```python
from build123d import *

# Parameters (mm, degrees)
SKETCH1_W           = 14
SKETCH1_H           = 10
SKETCH1_W_2         = 30
SKETCH1_H_2         = 30
BOSS_EXTRUDE1_DEPTH = 10
FILLET1_R           = 2


with BuildPart() as part:
    # Sketch1 → Boss-Extrude1 (new body)
    with BuildSketch(Plane.XY):
        with Locations((0, -5)):
            Rectangle(SKETCH1_W, SKETCH1_H)
        with Locations((0, 15)):
            Rectangle(SKETCH1_W_2, SKETCH1_H_2)
    extrude(amount=BOSS_EXTRUDE1_DEPTH)

    # Fillet1
    fillet1_edges = [part.edges().sort_by_distance(p)[0] for p in [
        (7, -10, 5),
        (-7, -10, 5),
        (-15, 0, 5),
        (-15, 30, 5),
        (15, 30, 5),
        (15, 0, 5),
    ]]
    fillet(fillet1_edges, radius=FILLET1_R)


solid = part.part
```
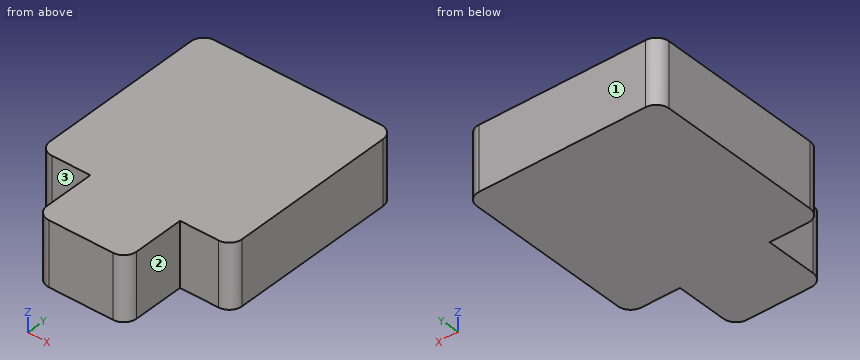
Check sheet for the modelled part. Datum: model origin and axes. Units: mm. Face numbers are marked on the shaded views. A direction names the side the tool comes from. Give positions to 0.01 mm unless a question says otherwise; leave off trailing zeros. Loops run counter-clockwise (first coordinate to the right, second up) from the corner with the lowest first, then second, coordinate; pieces in that order, holes last. Notation, with made-up numbers: (-15, 60.25) - (11, 60.25) arc R24 cw to (11, 70.25) - close; hole circle Ø3 at (4, 22). An arc over 180 degrees is marked (long way). One line per question, with ' | ' between items. Start each with the question number.
1. Gauge pin test, flat ends, axial feed: pin 1 Ø3 at (x, z) = (-9, 4) entering from -Y; pin 2 Ø6 at (x, y) = (-10.5, 14) entering from -Z; pin 3 Ø1.5 at (y, z) = (-2.5, 5) entering from -X; pin 4 Ø2.5 at (y, z) = (-5.5, 3) entering from +X. Record the tip position at first contact, or that the pin passes through.
2. Cross-section at B-B, the plane y = -4.5. Enter the section's corners in (x, z), plus the area to 3 significant figures.
3. Material ranges on line 1 along Y through (x, z) = (7.5, 6.5); line 2 along X through (y, z) = (-6, 3.5); line 3 along Y through (x, z) = (-6.75, 3.75), recorded low to high. Write a range as [from, to].
4. Cross-section at C-C, the plane x = 8.25. Enter the section's corners in (y, z).
5. Cross-section at A-A, the plane z = 4. Enter the section's corners in (x, y), plus the area to 3 significant figures.
6. Set-up check for the marked faces 1, 2 and 3: record each of +Z, -Z, +X, -X, +Y, -Y from which the full face is reachable in a straight line by a thin tool's end or side.
Check result:
1) pin 1: stops at y = 0 | pin 2: stops at z = 0 | pin 3: stops at x = -7 | pin 4: stops at x = 7
2) outline: (-7, 0) - (7, 0) - (7, 10) - (-7, 10) - close | area: 140 mm2
3) line 1: y = [0, 30] | line 2: x = [-7, 7] | line 3: y = [-8.97, 30]
4) outline: (0, 0) - (30, 0) - (30, 10) - (0, 10) - close
5) outline: (-15, 2) arc R2 ccw to (-13, 0) - (-7, 0) - (-7, -8) arc R2 ccw to (-5, -10) - (5, -10) arc R2 ccw to (7, -8) - (7, 0) - (13, 0) arc R2 ccw to (15, 2) - (15, 28) arc R2 ccw to (13, 30) - (-13, 30) arc R2 ccw to (-15, 28) - close | area: 1,030 mm2
6) face 1: +Z, -Z, +X, -X, +Y | face 2: +Z, -Z, +X, -Y | face 3: +Z, -Z, -X, -Y
